from build123d import *

# Parameters (mm, degrees)
BOSS_EXTRUDE1_DEPTH = 10
SKETCH2_R           = 2.5
CUT_EXTRUDE1_DEPTH  = 10
CIRPATTERN2_COUNT   = 4
CUT_EXTRUDE2_START  = 1
CUT_EXTRUDE2_DEPTH  = 6
CIRPATTERN3_COUNT   = 4


with BuildPart() as part:
    # Sketch1 → Boss-Extrude1 (new body)
    with BuildSketch(Plane(origin=(0, 0, 0), x_dir=(1, 0, 0), z_dir=(0, 1, 0))):
        Polygon((-48.197888799, 37.109268565), (-48.738098109, -40.767831949), (-48.738098109, -48.945710496), (-37.607816364, -48.945710496), (40.26928415, -49.485919806), (48.447162698, -49.485919806), (48.447162698, -38.355638061), (48.987372008, 39.521462453), (48.987372008, 47.699341001), (37.857090263, 47.699341001), (-40.020010251, 48.239550311), (-48.197888799, 48.239550311), align=None)
        Polygon((-40.033883465, 44.239550311), (-44.197888799, 44.239550311), (-44.197888799, 37.095395352), (-44.738098109, -40.781705162), (-44.738098109, -44.945710496), (-37.59394315, -44.945710496), (40.283157364, -45.485919806), (44.447162698, -45.485919806), (44.447162698, -38.341764848), (44.987372008, 39.535335666), (44.987372008, 43.699341001), (37.843217049, 43.699341001), align=None, mode=Mode.SUBTRACT)
    extrude(amount=BOSS_EXTRUDE1_DEPTH)

    # Sketch2 → Cut-Extrude1 (cut)
    with BuildSketch(Plane(origin=(0.332681132, 0, -47.959636197), x_dir=(-0.999975942033621, 0, -0.006936523190502626), z_dir=(0.006936523190502627, 0, -0.9999759420336211))):
        with Locations(Location((40.353662211, 5, 0), (0, 0, 270))):
            Circle(SKETCH2_R)
    cut_extrude1 = extrude(amount=-CUT_EXTRUDE1_DEPTH, mode=Mode.SUBTRACT)

    # CirPattern2: Cut-Extrude1 ×4 about axis
    cirpattern2_axis = Axis((0.12463695, 10, 0.623184748), (0, -1, 0))
    for i in range(1, CIRPATTERN2_COUNT):
        add(cut_extrude1.rotate(cirpattern2_axis, i * 360 / CIRPATTERN2_COUNT), mode=Mode.SUBTRACT)

    # Sketch6 → Cut-Extrude2 (cut)
    with BuildSketch(Plane(origin=(-0.341314401, 0, 49.20421667), x_dir=(0.999975942033621, 0, 0.006936523190502982), z_dir=(-0.006936523190502983, 0, 0.9999759420336211)).offset(CUT_EXTRUDE2_START)):
        with BuildLine():
            Line((40.611575584, 7.5), (-15.76739854, 7.5))
            ThreePointArc((-15.76739854, 7.5), (-18.26739854, 5), (-15.76739854, 2.5))
            Line((-15.76739854, 2.5), (40.611575584, 2.5))
            ThreePointArc((40.611575584, 2.5), (43.111575584, 5), (40.611575584, 7.5))
        make_face()
    cut_extrude2 = extrude(amount=-CUT_EXTRUDE2_DEPTH, mode=Mode.SUBTRACT)

    # CirPattern3: Cut-Extrude2 ×4 about axis
    cirpattern3_axis = Axis((0.12463695, 10, 0.623184748), (0, -1, 0))
    for i in range(1, CIRPATTERN3_COUNT):
        add(cut_extrude2.rotate(cirpattern3_axis, i * 360 / CIRPATTERN3_COUNT), mode=Mode.SUBTRACT)


solid = part.part
Here's how the part is built. I have some questions about the finished solid (model axes, mm). A direction names the side the tool comes from. Round coordinates to 2 decimals unless told otherwise and drop trailing zeros. Order: outer loops, then holes, each group sorted by start corner. A loop starts at its lowest first (then second) coordinate and runs counter-clockwise, first axis right, second up. Notation, with made-up numbers: (57, -20.5) -> (82, -20.5) arc R17 ccw to (82, -8.5) -> close; hole circle Ø6 at (36, 75). An arc over 180 degrees is marked (long way). Return JSON: item names as keys, results as strings.
Q1. If we mould it in two halves opening along Z, with no side actions, what happens to faces 4 (the flat face through (44.447, 5, 42)), 5 (the flat face through (47, 2.5, -11)), 6 (the flat face through (44, 5, 49.486))? For each: released by +Z, released by -Z, zero draft, split by the parting line, or undercut.
Filled sheet:
{"face 4": "undercut", "face 5": "undercut", "face 6": "released by +Z"}
Q2. I need wall thicknesses on line 1 along Y through (x, z) = (45, -21); line 2 along X through (y, z) = (2.25, 42); line 3 along X through (y, z) = (6, -35). Which ranges of each line are inside material? Lowest first, please. Write a range as from..to.
Filled sheet:
{"line 1": "y = 0..2.5, 7.5..10", "line 2": "x = -48.74..-44.74, 44.45..48.45", "line 3": "x = -48.21..-44.21"}
Q3. If we section it at D-D on z = -5: List the corners of the cut face in (x, y) for me.
Filled sheet:
{"outline": "(-48.42, 0) -> (-44.42, 0) -> (-44.42, 2.5) -> (-48.42, 2.5) -> close; (-48.42, 7.5) -> (-44.42, 7.5) -> (-44.42, 10) -> (-48.42, 10) -> close; (44.75, 0) -> (48.75, 0) -> (48.75, 2.5) -> (44.75, 2.5) -> close; (44.75, 7.5) -> (48.75, 7.5) -> (48.75, 10) -> (44.75, 10) -> close"}
Q4. If we section it at B-B on z = -30: List the corners of the cut face in (x, y) for me, plus the area to 3 significant figures.
Filled sheet:
{"outline": "(-48.25, 0) -> (-44.25, 0) -> (-44.25, 10) -> (-48.25, 10) -> close; (44.92, 0) -> (48.92, 0) -> (48.92, 2.5) -> (44.92, 2.5) -> close; (44.92, 7.5) -> (48.92, 7.5) -> (48.92, 10) -> (44.92, 10) -> close", "area": "60.0 mm^2"}
Q5. If we section it at A-A on y = 8.75: List the corners of the cut face in (x, z) for me.
Filled sheet:
{"outline": "(-48.74, 40.77) -> (-48.2, -37.11) -> (-48.2, -48.24) -> (-40.02, -48.24) -> (37.86, -47.7) -> (48.99, -47.7) -> (48.99, -39.52) -> (48.45, 38.36) -> (48.45, 49.49) -> (40.27, 49.49) -> (-37.61, 48.95) -> (-48.74, 48.95) -> close; hole (-44.74, 40.78) -> (-44.2, -37.1) -> (-44.2, -44.24) -> (-40.03, -44.24) -> (37.84, -43.7) -> (44.99, -43.7) -> (44.99, -39.54) -> (44.45, 38.34) -> (44.45, 45.49) -> (40.28, 45.49) -> (-37.59, 44.95) -> (-44.74, 44.95) -> close"}
Q6. If we section it at C-C on x = -9: List the corners of the cut face in (y, z) for me, plus the area to 3 significant figures.
Filled sheet:
{"outline": "(0, -48.02) -> (2.5, -48.02) -> (2.5, -44.02) -> (0, -44.02) -> close; (0, 45.14) -> (2.5, 45.14) -> (2.5, 49.14) -> (0, 49.14) -> close; (7.5, -48.02) -> (10, -48.02) -> (10, -44.02) -> (7.5, -44.02) -> close; (7.5, 45.14) -> (10, 45.14) -> (10, 49.14) -> (7.5, 49.14) -> close", "area": "40.0 mm^2"}
Q7. Which directions (+Z, -Z, +X, -X, +Y, -Y) give clear straight access to the entire face, cutting with the end or side of a thin tool? Please do faces 1 (the flat face through (12, 7.5, 47)), 2 (the flat face through (-48.198, 5, -43)), 3 (the flat face through (47, 7.5, -12)).
Filled sheet:
{"face 1": "+Z", "face 2": "-Z, -X, +Y, -Y", "face 3": "+X"}
Q8. For pin 1 Ø2 at (y, z) = (7, -41.5) entering from -X; pin 2 Ø3.5 at (x, y) = (43, 3) entering from -Z; pin 3 Ø1 at (x, y) = (-20, 8) entering from -Z, each with a flat end and sliding along its axis, tell me the tip position at first contact or that it passes through.
Filled sheet:
{"pin 1": "stops at x = -48.2", "pin 2": "stops at z = -47.7", "pin 3": "stops at z = -48.1"}
